from build123d import *

# Parameters (mm, degrees)
BOSS_EXTRUDE1_DEPTH = 4.5
FILLET1_R           = 0.3
LPATTERN1_START     = -4.5
LPATTERN1_DEPTH     = 9


# Read off the part's stored shape, not the designer's step: LPattern1
with BuildPart() as part:
    # Sketch1 → Boss-Extrude1 (new, symmetric)
    with BuildSketch(Plane.XY):
        Polygon((0, 0), (5, 0), (5, -2.08), (3.814834253, -2.08), (3.185165747, -3.81), (1.814834253, -3.81), (1.185165747, -2.08), (0, -2.08), align=None)
    extrude(amount=BOSS_EXTRUDE1_DEPTH, both=True)

    # Fillet1
    fillet1_edges = [part.edges().sort_by_distance(p)[0] for p in [
        (3.814834253, -2.08, 0),
        (3.185165747, -3.81, 0),
        (1.814834253, -3.81, 0),
        (1.185165747, -2.08, 0),
    ]]
    fillet(fillet1_edges, radius=FILLET1_R)

    # LPattern1 outline → LPattern1 (add)
    with BuildSketch(Plane.XY.offset(LPATTERN1_START)):
        with BuildLine():
            Line((5, -2.08), (5.975103486, -2.08))
            ThreePointArc((5.975103486, -2.08), (6.147176417, -2.134254387), (6.257011272, -2.277393957))
            Line((6.257011272, -2.277393957), (6.742988728, -3.612606043))
            ThreePointArc((6.742988728, -3.612606043), (6.852823583, -3.755745613), (7.024896514, -3.81))
            Line((7.024896514, -3.81), (7.975103486, -3.81))
            ThreePointArc((7.975103486, -3.81), (8.147176417, -3.755745613), (8.257011272, -3.612606043))
            Line((8.257011272, -3.612606043), (8.742988728, -2.277393957))
            ThreePointArc((8.742988728, -2.277393957), (8.852823583, -2.134254387), (9.024896514, -2.08))
            Line((9.024896514, -2.08), (10.975103486, -2.08))
            ThreePointArc((10.975103486, -2.08), (11.147176417, -2.134254387), (11.257011272, -2.277393957))
            Line((11.257011272, -2.277393957), (11.742988728, -3.612606043))
            ThreePointArc((11.742988728, -3.612606043), (11.852823583, -3.755745613), (12.024896514, -3.81))
            Line((12.024896514, -3.81), (12.975103486, -3.81))
            ThreePointArc((12.975103486, -3.81), (13.147176417, -3.755745613), (13.257011272, -3.612606043))
            Line((13.257011272, -3.612606043), (13.742988728, -2.277393957))
            ThreePointArc((13.742988728, -2.277393957), (13.852823583, -2.134254387), (14.024896514, -2.08))
            Line((14.024896514, -2.08), (15.975103486, -2.08))
            ThreePointArc((15.975103486, -2.08), (16.147176417, -2.134254387), (16.257011272, -2.277393957))
            Line((16.257011272, -2.277393957), (16.742988728, -3.612606043))
            ThreePointArc((16.742988728, -3.612606043), (16.852823583, -3.755745613), (17.024896514, -3.81))
            Line((17.024896514, -3.81), (17.975103486, -3.81))
            ThreePointArc((17.975103486, -3.81), (18.147176417, -3.755745613), (18.257011272, -3.612606043))
            Line((18.257011272, -3.612606043), (18.742988728, -2.277393957))
            ThreePointArc((18.742988728, -2.277393957), (18.852823583, -2.134254387), (19.024896514, -2.08))
            Line((19.024896514, -2.08), (20.975103486, -2.08))
            ThreePointArc((20.975103486, -2.08), (21.147176417, -2.134254387), (21.257011272, -2.277393957))
            Line((21.257011272, -2.277393957), (21.742988728, -3.612606043))
            ThreePointArc((21.742988728, -3.612606043), (21.852823583, -3.755745613), (22.024896514, -3.81))
            Line((22.024896514, -3.81), (22.975103486, -3.81))
            ThreePointArc((22.975103486, -3.81), (23.147176417, -3.755745613), (23.257011272, -3.612606043))
            Line((23.257011272, -3.612606043), (23.742988728, -2.277393957))
            ThreePointArc((23.742988728, -2.277393957), (23.852823583, -2.134254387), (24.024896514, -2.08))
            Line((24.024896514, -2.08), (25, -2.08))
            Line((25, -2.08), (25, 0))
            Line((25, 0), (5, 0))
            Line((5, 0), (5, -2.08))
        make_face()
    extrude(amount=LPATTERN1_DEPTH)


solid = part.part
Verification items for the finished model (mm, model axes). A direction names the side the tool comes from. Give positions to 0.01 mm unless a question says otherwise; leave off trailing zeros. Write each loop counter-clockwise with the first axis right and the second up, starting at its lowest first coordinate (ties: lowest second). Pieces come first, ordered by that corner, then holes. Notation, with made-up numbers: M -5.75,59 L 24.25,59 A27 cw 24.25,95 Z; hole C 28.5,54.25 d9. An arc over 180 degrees is marked long. Put each result on its own line as item: value. Start each with the question number.
1. Section check A-A (x = 8.5). Record the cut outline in (y, z) (3 decimals).
2. Draft check along X on faces 1 (the face through (0, -1, 0)), 2 (the face through (24.5, -2.08, -0.1)), 3 (the face through (18.5, -2.95, -0.06)). Enter one of: +X half, -X half, draft (parallel to the pull), parting line (faces both ways), or undercut.
3. Set-up check for faces 4 (the face through (7.5, -3.81, -0.1)), 5 (the face through (0.5, -2.08, 0.1)), 6 (the face through (15, -2.08, 0)): record each of +Z, -Z, +X, -X, +Y, -Y from which the full face is reachable in a straight line by a thin tool's end or side.
4. Scan lines: line 1 along X through (y, z) = (-3.6, 3); line 2 along X through (y, z) = (-2.5, 3.25); line 3 along Y through (x, z) = (21, -3). Record each from-to range of solid material in increasing order. Write a range as [from, to].
5. Go/stop test with flat-tipped pins: pin 1 Ø1 at (y, z) = (-3, 0.5) entering from -X; pin 2 Ø1.1 at (x, z) = (0.5, -0.5) entering from -Y; pin 3 Ø1 at (x, z) = (13.5, -2.5) entering from -Y. Record where each tip stops, or that it passes through.
Answer list:
1. outline: M -2.945,-4.5 L 0,-4.5 L 0,4.5 L -2.945,4.5 Z
2. face 1: -X half
2. face 2: draft
2. face 3: undercut
3. face 4: +Z, -Z, +X, -X, -Y
3. face 5: +Z, -Z, -X, -Y
3. face 6: +Z, -Z, -Y
4. line 1: [1.74, 3.26], [6.74, 8.26], [11.74, 13.26], [16.74, 18.26], [21.74, 23.26]
4. line 2: [1.34, 3.66], [6.34, 8.66], [11.34, 13.66], [16.34, 18.66], [21.34, 23.66]
4. line 3: [-2.08, 0]
5. pin 1: x = 1.34
5. pin 2: y = -2.09
5. pin 3: y = -3.81
